```python
from build123d import *

# Parameters (mm, degrees)
F0_R          = 57.9269385224
F0_R_2        = 45.238930614
F0_R_3        = 10.232456426
F0_R_4        = 9.9260337363
F0_R_5        = 10.3400506536
F1_DEPTH      = 12.7
F2_DEPTH      = 12.7
F3_R          = 44.8601198224
F4_DEPTH      = 6.35
F5_R          = 44.7159015694
F6_DEPTH      = 6.35
F8_DEPTH      = 6.35
F10_DEPTH     = 6.35
F11_R         = 10.0879812564
F11_R_2       = 10.1077702508
F11_R_3       = 10.130036121
F12_DEPTH     = 6.35
F16_T4_DEPTH  = 143.3938123808
F16_T11_DEPTH = 146.5521785494
F16_T18_DEPTH = 143.0711301992


# Not quite as in the source:
# - a fillet or chamfer that OpenCascade refuses, or shapes differently, is made with other operations: its cross-section is extruded or revolved along the edge and cut away or added


with BuildPart() as f1:
    # F0 (on Front) → F1 (new body)
    with BuildSketch(Plane.XZ):
        Circle(F0_R)
        Circle(F0_R_2, mode=Mode.SUBTRACT)
        Circle(F0_R_2)
        with Locations((-26.1295642704, -15.3669575229)):
            Circle(F0_R_3, mode=Mode.SUBTRACT)
        Polygon((-12.544834055, -34.5090515912), (0, -5.3877583705), (12.6424450427, -34.5090515912), align=None, mode=Mode.SUBTRACT)
        with Locations((26.1333119124, -15.1850637048)):
            Circle(F0_R_4, mode=Mode.SUBTRACT)
        Polygon((-36.0336452723, 4.8764180392), (-24.01153557, 26.9035063684), (-4.5260344632, 1.7700339667), align=None, mode=Mode.SUBTRACT)
        Polygon((36.1581519246, 4.842239432), (4.4649434276, 1.758374623), (24.0084677935, 26.875147596), align=None, mode=Mode.SUBTRACT)
        with Locations((0, 29.5979101211)):
            Circle(F0_R_5, mode=Mode.SUBTRACT)
        with Locations((0, 29.5979101211)):
            Circle(F0_R_5)
        Polygon((-4.5260344632, 1.7700339667), (-24.01153557, 26.9035063684), (-36.0336452723, 4.8764180392), align=None)
        with Locations((-26.1295642704, -15.3669575229)):
            Circle(F0_R_3)
        Polygon((12.6424450427, -34.5090515912), (0, -5.3877583705), (-12.544834055, -34.5090515912), align=None)
        with Locations((26.1333119124, -15.1850637048)):
            Circle(F0_R_4)
        Polygon((24.0084677935, 26.875147596), (4.4649434276, 1.758374623), (36.1581519246, 4.842239432), align=None)
    extrude(amount=F1_DEPTH)

    # F2 (add): a face of the model
    f2_faces = [f1.faces().sort_by_distance(p)[0] for p in [
        (0, 0, 0),
    ]]
    extrude(f2_faces, amount=F2_DEPTH)

    # F3 (on face) → F4 (cut)
    with BuildSketch(Plane.XZ.offset(12.7)):
        Circle(F3_R)
    extrude(amount=-F4_DEPTH, mode=Mode.SUBTRACT)

    # F5 (on face) → F6 (cut)
    with BuildSketch(Plane(origin=(0, 12.7, 0), x_dir=(-1, 0, 0), z_dir=(0, 1, 0))):
        Circle(F5_R)
    extrude(amount=-F6_DEPTH, mode=Mode.SUBTRACT)

    # F7 (on face) → F8 (join)
    with BuildSketch(Plane(origin=(0, 6.35, 0), x_dir=(-1, 0, 0), z_dir=(0, 1, 0))):
        Polygon((0.1139463857, -15.4419038445), (-13.0555815995, 7.0367623121), (-26.1111631989, -15.4419038445), align=None)
        Polygon((0.1139463857, -15.4419038445), (13.1695279852, 7.0367623121), (-13.0555815995, 7.0367623121), align=None)
        Polygon((13.1695279852, 7.0367623121), (0, 29.5154284686), (-13.0555815995, 7.0367623121), align=None)
        Polygon((26.3390559703, -15.4419038445), (13.1695279852, 7.0367623121), (0.1139463857, -15.4419038445), align=None)
    extrude(amount=F8_DEPTH)

    # F9 (on face) → F10 (cut)
    with BuildSketch(Plane(origin=(0, 12.7, 0), x_dir=(-1, 0, 0), z_dir=(0, 1, 0))):
        Polygon((12.9840383306, 6.3451784663), (-12.7162076533, 6.3451784663), (0, -15.0037035346), align=None)
    extrude(amount=-F10_DEPTH, mode=Mode.SUBTRACT)

    # F11 (on face) → F12 (join)
    with BuildSketch(Plane.XZ.offset(6.35)):
        with Locations((0.4030804266, 29.4006802142)):
            Circle(F11_R)
        with Locations((26.4969747514, -15.3808789328)):
            Circle(F11_R_2)
        with Locations((-25.7336739451, -15.2944726869)):
            Circle(F11_R_3)
        Polygon((0.1468855771, -31.126530841), (30.5121447891, 17.0675422996), (-29.6086445451, 17.0675422996), align=None)
    extrude(amount=F12_DEPTH)

    # F13: fillet of radius 10.922 on 1 edges, made by hand

    # F13_s1 → F13_t2 (revolve, cut)
    with BuildSketch(Plane.XY.offset(29.4006802142)):
        with BuildLine():
            ThreePointArc((10.491061683, -6.35), (6.4607923392, -10.9765180328), (0.5720445946, -12.7))
            Line((0.5720445946, -12.7), (10.491061683, -12.7))
            Line((10.491061683, -12.7), (10.491061683, -6.35))
        make_face()
    revolve(axis=Axis((0.4030804266, -12.7, 29.4006802142), (0, -1, 0)), mode=Mode.SUBTRACT)

    # F14: fillet of radius 11.049 on 1 edges, made by hand

    # F14_s1 → F14_t2 (revolve, cut)
    with BuildSketch(Plane.XY.offset(-15.2944726869)):
        with BuildLine():
            ThreePointArc((-15.6036378241, -6.35), (-19.6807421254, -10.9783697257), (-25.6036278241, -12.7))
            Line((-25.6036278241, -12.7), (-15.6036378241, -12.7))
            Line((-15.6036378241, -12.7), (-15.6036378241, -6.35))
        make_face()
    revolve(axis=Axis((-25.7336739451, -12.7, -15.2944726869), (0, -1, 0)), mode=Mode.SUBTRACT)

    # F15: fillet of radius 11.049 on 1 edges, made by hand

    # F15_s1 → F15_t2 (revolve, cut)
    with BuildSketch(Plane.XY.offset(-15.3808789328)):
        with BuildLine():
            ThreePointArc((36.6047450022, -6.35), (32.5276407009, -10.9783697257), (26.6047550022, -12.7))
            Line((26.6047550022, -12.7), (36.6047450022, -12.7))
            Line((36.6047450022, -12.7), (36.6047450022, -6.35))
        make_face()
    revolve(axis=Axis((26.4969747514, -12.7, -15.3808789328), (0, -1, 0)), mode=Mode.SUBTRACT)

    # F16: chamfer of 16.6624 x 6.3960960974 on 3 edges, made by hand


with BuildPart() as f16_tool2:
    # F16_s3 → F16_t4 (new body)
    with BuildSketch(Plane(origin=(-37.0340982639, 0, -58.7784885341), x_dir=(0, 1, 0), z_dir=(0.5330752718, 0, 0.8460678191))):
        Polygon((-6.3039039026, -16.7170590485), (-12.7, -0.0546590485), (-12.7, -16.7170590485), align=None)
    extrude(amount=F16_T4_DEPTH)

    split(bisect_by=Plane.XZ.offset(6.35), keep=Keep.TOP)

    split(bisect_by=Plane.XY.offset(17.0675422996), keep=Keep.BOTTOM)

    split(bisect_by=Plane(origin=(-13.8075741275, 0, -8.5249421991), x_dir=(0, 1, 0), z_dir=(0.8508879508, 0, 0.5253472139)), keep=Keep.TOP)


with BuildPart() as f1_1:
    add(f1.part)

    # F16_t1: cut F16_tool2
    add(f16_tool2.part, mode=Mode.SUBTRACT)


with BuildPart() as f16_tool9:
    # F16_s10 → F16_t11 (new body)
    with BuildSketch(Plane.YZ.offset(73.7278393967)):
        Polygon((-6.3039039026, 17.0675422996), (-12.7, 0.4051422996), (-12.7, 17.0675422996), align=None)
    extrude(amount=-F16_T11_DEPTH)

    split(bisect_by=Plane.XZ.offset(6.35), keep=Keep.TOP)

    split(bisect_by=Plane(origin=(14.1437656916, 0, -8.9114507961), x_dir=(0, 1, 0), z_dir=(-0.8460678191, 0, 0.5330752718)), keep=Keep.TOP)

    split(bisect_by=Plane(origin=(-13.8075741275, 0, -8.5249421991), x_dir=(0, 1, 0), z_dir=(0.8508879508, 0, 0.5253472139)), keep=Keep.TOP)


with BuildPart() as f1_2:
    add(f1_1.part)

    # F16_t8: cut F16_tool9
    add(f16_tool9.part, mode=Mode.SUBTRACT)


with BuildPart() as f16_tool16:
    # F16_s17 → F16_t18 (new body)
    with BuildSketch(Plane(origin=(-38.5043151766, 0, 62.3641983265), x_dir=(0, 1, 0), z_dir=(0.5253472139, 0, -0.8508879508))):
        Polygon((-6.3039039026, -16.2272530881), (-12.7, 0.4351469119), (-12.7, -16.2272530881), align=None)
    extrude(amount=F16_T18_DEPTH)

    split(bisect_by=Plane.XZ.offset(6.35), keep=Keep.TOP)

    split(bisect_by=Plane(origin=(14.1437656916, 0, -8.9114507961), x_dir=(0, 1, 0), z_dir=(-0.8460678191, 0, 0.5330752718)), keep=Keep.TOP)

    split(bisect_by=Plane.XY.offset(17.0675422996), keep=Keep.BOTTOM)


with BuildPart() as f1_3:
    add(f1_2.part)

    # F16_t15: cut F16_tool16
    add(f16_tool16.part, mode=Mode.SUBTRACT)


solid = f1_3.part
```
CAD build for the part. Positions are in the model's coordinates, mm. A direction names the side the tool comes from. Round coordinates to 2 decimals unless told otherwise and drop trailing zeros. Write each loop counter-clockwise with the first axis right and the second up, starting at its lowest first coordinate (ties: lowest second). Pieces come first, ordered by that corner, then holes. Notation, with made-up numbers: (-17.75, 77.25) -> (22.25, 77.25) arc R23 ccw to (22.25, 97.25) -> close; hole circle Ø3 at (-26, 10.5). An arc over 180 degrees is marked (long way). Answer in a Markdown table with one row per item. Add a question column.
Item 1: Saw through at B-B, the plane z = 3. Write the cut outline in (x, y), then the cut area to 3 significant figures.
Item 2: Drop flat-ended pins along their axis: pin 1 Ø1.9 at (x, y) = (-11.5, 10.5) entering from -Z; pin 2 Ø3 at (x, y) = (19.5, 9.5) entering from +Z; pin 3 Ø2 at (x, y) = (6, 2.5) entering from +Z. Give the stop position or say it passes through.
Item 3: Mould opens along Z. For faces 1 (the face through (-12.56, -0.18, -56.55)), 2 (the face through (-6.4, 9.57, -4.48)), 3 (the face through (30, -12.7, -34)) say: pulls with the +Z half, pulls with the -Z half, needs draft (parallel to the pull), parting line crosses it, or undercut.
Item 4: Saw through at D-D, the plane z = -40.5. Write the cut outline in (x, y).
Item 5: Drill centre lines: line 1 (Z direction, x = 0, y = 8.75); line 2 (Z direction, x = -20.5, y = 6.5); line 3 (X direction, y = 9.5, z = 12). Where is each one in solid material? Low to high. Write a range as from..to.
Item 6: Saw through at C-C, the plane x = -49. Write the cut outline in (y, z), then the cut area to 3 significant figures.
Item 7: Saw through at A-A, the plane y = 9. Write the cut outline in (x, z), then the cut area to 3 significant figures.
Item 8: Which spindle directions (+Z, -Z, +X, -X, +Y, -Y) get a long thin tool onto all of the face, cutting with end or side? Do faces 4 (the face through (0, 9, -15.442)), 5 (the face through (0, 12.7, 7)), 6 (the face through (-21, -6.35, 1)). Say none if no direction does.
Findings below:
| question | item | result |
|---|---|---|
| 1 | outline | (-57.85, -12.7) -> (-44.76, -12.7) -> (-44.76, -6.35) -> (-20.78, -6.35) -> (-4.39, -11.7) -> (5.02, -11.7) -> (21.51, -6.35) -> (44.76, -6.35) -> (44.76, -12.7) -> (57.85, -12.7) -> (57.85, 12.7) -> (44.62, 12.7) -> (44.62, 6.35) -> (15.4, 6.35) -> (15.4, 12.7) -> (10.72, 12.7) -> (10.72, 6.35) -> (-10.95, 6.35) -> (-10.95, 12.7) -> (-15.53, 12.7) -> (-15.53, 6.35) -> (-44.62, 6.35) -> (-44.62, 12.7) -> (-57.85, 12.7) -> close |
| 1 | area | 2,000 mm^2 |
| 2 | pin 1 | stops at z = -56.96 |
| 2 | pin 2 | stops at z = 55.06 |
| 2 | pin 3 | stops at z = 57.71 |
| 3 | face 1 | parting line crosses it |
| 3 | face 2 | undercut |
| 3 | face 3 | needs draft |
| 4 | outline | (-41.42, -12.7) -> (-19.29, -12.7) -> (-19.29, -6.35) -> (19.29, -6.35) -> (19.29, -12.7) -> (41.42, -12.7) -> (41.42, 12.7) -> (18.95, 12.7) -> (18.95, 6.35) -> (-18.95, 6.35) -> (-18.95, 12.7) -> (-41.42, 12.7) -> close |
| 5 | line 1 | z = -57.93..-44.72, -15.44..-15, 6.35..29.52, 44.72..57.93 |
| 5 | line 2 | z = -54.18..-39.74, -15.44..-5.48, 39.74..54.18 |
| 5 | line 3 | x = -56.67..-43.08, -10.26..10.17, 43.08..56.67 |
| 6 | outline | (-12.7, -30.9) -> (12.7, -30.9) -> (12.7, 30.9) -> (-12.7, 30.9) -> close |
| 6 | area | 1,570 mm^2 |
| 7 | outline | circle Ø115.85 at (0, 0); (-26.34, -15.44) -> (26.11, -15.44) -> (0, 29.52) -> close; hole circle Ø89.43 at (0, 0); hole (-12.98, 6.35) -> (0, -15) -> (12.72, 6.35) -> close |
| 7 | area | 5,160 mm^2 |
| 8 | face 4 | +Y |
| 8 | face 5 | +Z, -Z, +X, -X, +Y |
| 8 | face 6 | -Y |
